from build123d import *

# Parameters (mm, degrees)
F1_DEPTH  = 10
F0_W      = 7.5
F0_H      = 2.5
F2_DEPTH  = 9
F3_DEPTH  = 2
F5_R      = 4
F6_DEPTH  = 8
F7_DEPTH  = 2
F9_D      = 4.5
F9_DEPTH  = 29.101
F10_DEPTH = 1


with BuildPart() as f1:
    # F0 (on Front) → F1 (new body, symmetric)
    with BuildSketch(Plane.XZ):
        Polygon((0, 26.6), (0, 0), (40.5, 0), (40.5, 0.8176856209), (40.5, 2.4204463698), (40.5, 26.6), (40.5, 29.1), (40.5, 36.1), (0, 36.1), (0, 29.1), align=None)
    extrude(amount=F1_DEPTH, both=True)

    # F0 (on Front) → F2 (join, symmetric)
    with BuildSketch(Plane.XZ):
        with Locations((-3.75, 27.85)):
            Rectangle(F0_W, F0_H)
        with Locations((44.25, 27.85)):
            Rectangle(F0_W, F0_H)
    extrude(amount=F2_DEPTH, both=True)

    # F0 (on Front) → F3 (join, symmetric)
    with BuildSketch(Plane.XZ):
        Polygon((40.5, 2.4204463698), (40.5, 0.8176856209), (44.8900647461, 1.6190659953), align=None)
    extrude(amount=F3_DEPTH, both=True)

    # F5 (on plane+point) → F6 (join, through all)
    with BuildSketch(Plane.XY.offset(44.1)):
        with Locations((30.1, 0)):
            Circle(F5_R)
    extrude(amount=-F6_DEPTH)

    # F5 (on plane+point) → F7 (join)
    with BuildSketch(Plane.XY.offset(44.1)):
        with BuildLine():
            ThreePointArc((32.55, 16.95), (29.8633773569, 14.5114533581), (27.6957063471, 17.4210329401))
            Line((27.6957063471, 17.4210329401), (25.2356786223, 4.8643213777))
            Line((25.2356786223, 4.8643213777), (12.6789670858, 2.404293658))
            ThreePointArc((12.6789670858, 2.404293658), (14.7069954014, 1.8916303338), (15.6, 0))
            ThreePointArc((15.6, 0), (14.7069954014, -1.8916303338), (12.6789670858, -2.404293658))
            Line((12.6789670858, -2.404293658), (25.2356786223, -4.8643213777))
            Line((25.2356786223, -4.8643213777), (27.6957063471, -17.4210329401))
            ThreePointArc((27.6957063471, -17.4210329401), (29.8633773569, -14.5114533581), (32.55, -16.95))
            ThreePointArc((32.55, -16.95), (32.5385466419, -17.1866226431), (32.5042936529, -17.4210329401))
            Line((32.5042936529, -17.4210329401), (34.9643213777, -4.8643213777))
            Line((34.9643213777, -4.8643213777), (47.5210328982, -2.4042936611))
            ThreePointArc((47.5210328982, -2.4042936611), (44.6, 8.2e-09), (47.5210329142, 2.404293658))
            Line((47.5210329142, 2.404293658), (34.9643213777, 4.8643213777))
            Line((34.9643213777, 4.8643213777), (32.5042935187, 17.4210336249))
            ThreePointArc((32.5042935187, 17.4210336249), (32.5385466082, 17.1866229903), (32.55, 16.95))
        make_face()
        with Locations((30.1, 0)):
            Circle(F5_R, mode=Mode.SUBTRACT)
        with BuildLine():
            ThreePointArc((32.5042935187, 17.4210336249), (30.0999996511, 19.4), (27.6957063471, 17.4210329401))
            ThreePointArc((27.6957063471, 17.4210329401), (29.8633773569, 14.5114533581), (32.55, 16.95))
            ThreePointArc((32.55, 16.95), (32.5385466082, 17.1866229903), (32.5042935187, 17.4210336249))
        make_face()
        with BuildLine():
            ThreePointArc((49.5, 0), (48.9416303338, 1.5569954014), (47.5210329142, 2.404293658))
            ThreePointArc((47.5210329142, 2.404293658), (44.6, 8.2e-09), (47.5210328982, -2.4042936611))
            ThreePointArc((47.5210328982, -2.4042936611), (48.9416303286, -1.5569954077), (49.5, 0))
        make_face()
        with BuildLine():
            ThreePointArc((32.55, -16.95), (29.8633773569, -14.5114533581), (27.6957063471, -17.4210329401))
            ThreePointArc((27.6957063471, -17.4210329401), (30.1, -19.4), (32.5042936529, -17.4210329401))
            ThreePointArc((32.5042936529, -17.4210329401), (32.5385466419, -17.1866226431), (32.55, -16.95))
        make_face()
        with BuildLine():
            ThreePointArc((15.6, 0), (14.7069954014, 1.8916303338), (12.6789670858, 2.404293658))
            ThreePointArc((12.6789670858, 2.404293658), (10.7, 0), (12.6789670858, -2.404293658))
            ThreePointArc((12.6789670858, -2.404293658), (14.7069954014, -1.8916303338), (15.6, 0))
        make_face()
        with Locations((30.1, 0)):
            Circle(F5_R)
    extrude(amount=-F7_DEPTH)

    # F9 (through all, one way)
    with BuildSketch(Plane.XY.offset(29.1)):
        with Locations((-5, 5), (-5, -5), (45.5, 5), (45.5, -5)):
            Circle(F9_D / 2)
    extrude(amount=-F9_DEPTH, mode=Mode.SUBTRACT)

    # F8 (on face) → F10 (join)
    with BuildSketch(Plane.XY.offset(29.1)):
        with BuildLine():
            Line((0, -1), (0, 1))
            Line((0, 1), (-3, 1))
            ThreePointArc((-3, 1), (-3.7071067812, 0.7071067812), (-4, 0))
            ThreePointArc((-4, 0), (-3.7071067812, -0.7071067812), (-3, -1))
            Line((-3, -1), (0, -1))
        make_face()
        with BuildLine():
            Line((43.5, 1), (40.5, 1))
            Line((40.5, 1), (40.5, -1))
            Line((40.5, -1), (43.5, -1))
            ThreePointArc((43.5, -1), (44.2071067812, -0.7071067812), (44.5, 0))
            ThreePointArc((44.5, 0), (44.2071067812, 0.7071067812), (43.5, 1))
        make_face()
    extrude(amount=F10_DEPTH)


solid = f1.part
Input: part model. Units: mm. Frame: model coordinates. A direction names the side the tool comes from. Round coordinates to 2 decimals unless told otherwise and drop trailing zeros. Order: outer loops, then holes, each group sorted by start corner. A loop starts at its lowest first (then second) coordinate and runs counter-clockwise, first axis right, second up. Notation, with made-up numbers: (66.25, 28.25) - (87.25, 28.25) arc R19 cw to (87.25, 33.25) - close; hole circle Ø9 at (-8.75, 65). An arc over 180 degrees is marked (long way). Use a Markdown table: item, result.
1. Material intervals for probe 1 along Y at (x, z) = (45.5, 28.1); probe 2 along Z at (x, y) = (41, -1.5); probe 3 along Z at (x, y) = (21, 1), sorted ascending.
Evaluation:
| item | result |
|---|---|
| probe 1 | -9 to -7.25, -2.75 to 2.75, 7.25 to 9 |
| probe 2 | 0.91 to 2.33, 26.6 to 29.1, 42.1 to 44.1 |
| probe 3 | 0 to 36.1, 42.1 to 44.1 |
2. Access query for faces 5 (the face through (-4, -9, 28)), 6 (the face through (33.752, 11.055, 43.114)), 7 (the face through (41.155, -3.652, 43.114)). Directions: +Z, -Z, +X, -X, +Y, -Y. A direction counts if a zero-diameter tool reaches every point of the face in a straight line with its end or side. Return the directions, or none.
Evaluation:
| item | result |
|---|---|
| face 5 | +Z, -Z, -X, -Y |
| face 6 | +Z, +X, +Y |
| face 7 | +Z, +X, -Y |
3. First-contact query: pin 1 (1 mm diameter, centred on x = 30, z = 35, fed in from -Y); pin 2 (5 mm diameter, centred on x = -5, y = 5, fed in from +Z); pin 3 (1 mm diameter, centred on x = 41.5, z = 21.5, fed in from -Y); pin 4 (0.8 mm diameter, centred on x = 43, z = 1.5, fed in from -Y). Flat tips, straight axial feed; report the tip coordinate or a pass-through.
Evaluation:
| item | result |
|---|---|
| pin 1 | y = -10 |
| pin 2 | z = 29.1 |
| pin 3 | through |
| pin 4 | y = -2 |
4. Section C-C on z = 14.5. Return the cut outline in (x, y), then the cut area to 3 significant figures.
Evaluation:
| item | result |
|---|---|
| outline | (0, -10) - (40.5, -10) - (40.5, 10) - (0, 10) - close |
| area | 810 mm^2 |
5. Section D-D on x = 4. Return the cut outline in (y, z), then the cut area to 3 significant figures.
Evaluation:
| item | result |
|---|---|
| outline | (-10, 0) - (10, 0) - (10, 36.1) - (-10, 36.1) - close |
| area | 722 mm^2 |
6. Section A-A on x = -5. Return the cut outline in (y, z).
Evaluation:
| item | result |
|---|---|
| outline | (-9, 26.6) - (-7.25, 26.6) - (-7.25, 29.1) - (-9, 29.1) - close; (-2.75, 26.6) - (2.75, 26.6) - (2.75, 29.1) - (-2.75, 29.1) - close; (7.25, 26.6) - (9, 26.6) - (9, 29.1) - (7.25, 29.1) - close |
7. Section B-B on x = 30.1. Return the cut outline in (y, z), then the cut area to 3 significant figures.
Evaluation:
| item | result |
|---|---|
| outline | (-19.4, 42.1) - (-4, 42.1) - (-4, 36.1) - (-10, 36.1) - (-10, 0) - (10, 0) - (10, 36.1) - (4, 36.1) - (4, 42.1) - (19.4, 42.1) - (19.4, 44.1) - (-19.4, 44.1) - close |
| area | 848 mm^2 |
8. Mould query, pull axis Z, two halves, no side actions, for faces 1 (the face through (27, -3, 42.1)), 2 (the face through (21, 0, 36.1)), 3 (the face through (0, 0, 18)), 4 (the face through (-4, 0, 26.6)). Classes: +Z half, -Z half, draft (parallel to the pull), parting line (faces both ways), or undercut.
Evaluation:
| item | result |
|---|---|
| face 1 | undercut |
| face 2 | undercut |
| face 3 | draft |
| face 4 | -Z half |
